Source: three-view drawing plus pictorial views. Frame: mm from the lowest corner of the part. A direction names the side the tool comes from. Give positions to 0.01 mm unless a question says otherwise; leave off trailing zeros. Order: outer loops, then holes, each group sorted by start corner. A loop starts at its lowest first (then second) coordinate and runs counter-clockwise, first axis right, second up.
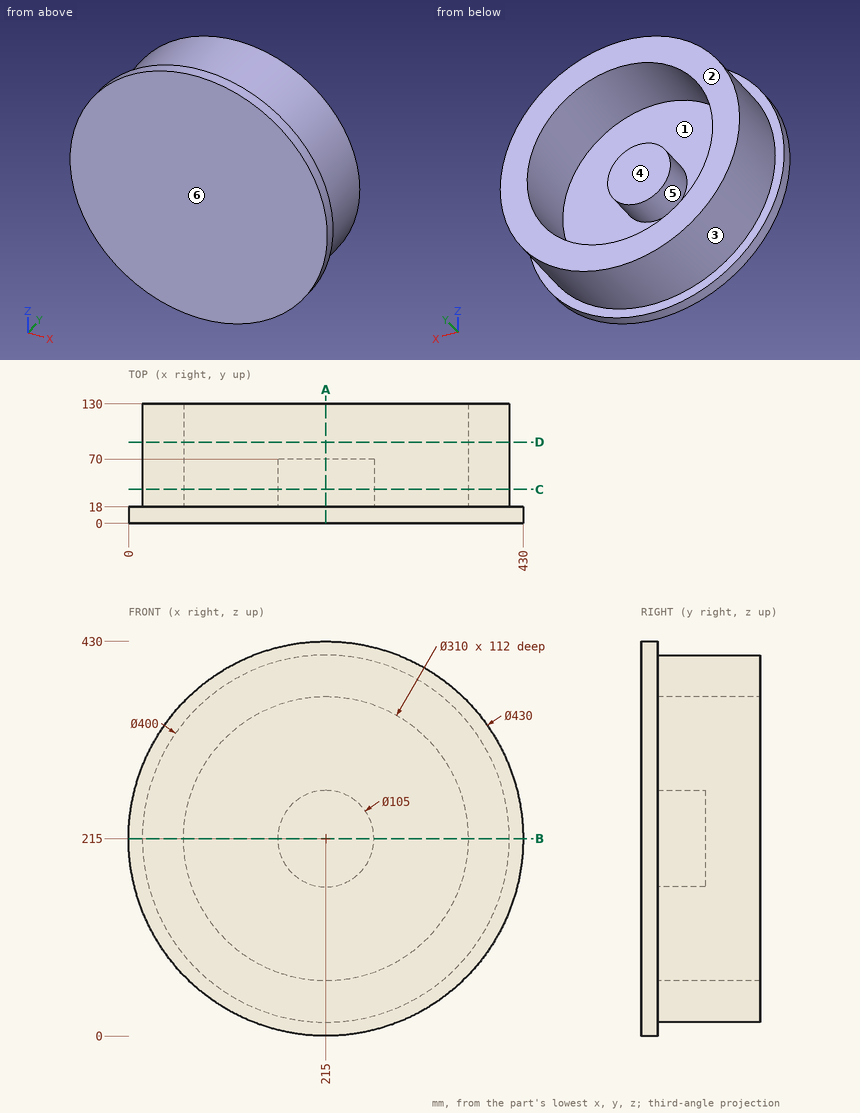
1) Section query C-C on y = 37. Output: boundary loops of the cut face in (x, z).
Checks:
outline: circle Ø400 at (215, 215); circle Ø105 at (215, 215); hole circle Ø310 at (215, 215)
2) Section query B-B on z = 215. Output: boundary loops of the cut face in (x, y), and give its area (3 significant figures).
Checks:
outline: (0, 0) - (430, 0) - (430, 18) - (415, 18) - (415, 130) - (370, 130) - (370, 18) - (267.5, 18) - (267.5, 70) - (162.5, 70) - (162.5, 18) - (60, 18) - (60, 130) - (15, 130) - (15, 18) - (0, 18) - close
area: 23,300 mm2
3) Reachability of the marked faces 1 and 2 from +Z, -Z, +X, -X, +Y, -Y: full face, straight path, thin tool, end or side. Return the list, or none.
Checks:
face 1: +Y
face 2: +Z, -Z, +X, -X, +Y
4) Section query D-D on y = 88.5. Output: boundary loops of the cut face in (x, z).
Checks:
outline: circle Ø400 at (215, 215); hole circle Ø310 at (215, 215)
5) Section query A-A on x = 215. Output: boundary loops of the cut face in (y, z), and give its area (3 significant figures).
Checks:
outline: (0, 0) - (18, 0) - (18, 15) - (130, 15) - (130, 60) - (18, 60) - (18, 162.5) - (70, 162.5) - (70, 267.5) - (18, 267.5) - (18, 370) - (130, 370) - (130, 415) - (18, 415) - (18, 430) - (0, 430) - close
area: 23,300 mm2
6) First-contact query: pin 1 Ø3 at (y, z) = (24.5, 103.5) entering from +X; pin 2 Ø1.5 at (y, z) = (80.5, 52) entering from +X; pin 3 Ø12 at (x, y) = (349, 56) entering from -Z (3 decimals). Flat tips, straight axial feed; report the tip coordinate or a pass-through.
Checks:
pin 1: stops at x = 382.03
pin 2: stops at x = 331.94
pin 3: stops at z = 61.325
7) Ray query, L1, parallel to Z at x = 215, y = 67; L2, parallel to Z at x = 215, y = 101.5. Return the intervals inside material, ascending.
Checks:
L1: z = 15 to 60, 162.5 to 267.5, 370 to 415
L2: z = 15 to 60, 370 to 415
8) Pull-direction query (Z, two-part tool) for the marked faces 3, 4, 5 and 6; classes: +Z half, -Z half, draft (parallel to the pull), parting line (faces both ways), or undercut.
Checks:
face 3: parting line
face 4: undercut
face 5: undercut
face 6: draft
